The listing builds one solid part. Answer for the finished solid, in the listing's coordinates (mm). A direction names the side the tool comes from. Coordinates: 2 decimals unless noted, no trailing zeros. Order: outer loops, then holes, each group sorted by start corner. A loop starts at its lowest first (then second) coordinate and runs counter-clockwise, first axis right, second up.
```python
from build123d import *

# Parameters (mm, degrees)
CUT_EXTRUDE1_DEPTH = 1.4
SKETCH5_R          = 1.15
CUT_EXTRUDE2_DEPTH = 22.529180779
CUT_EXTRUDE3_DEPTH = 1.475


with BuildPart() as part:
    # Sketch1 → Revolve1 (revolve)
    with BuildSketch(Plane(origin=(0, 0, 0), x_dir=(0, 0, -1), z_dir=(1, 0, 0)), mode=Mode.PRIVATE) as revolve1_sk:
        with BuildLine():
            Line((-1.8375, 0), (1.8375, 0))
            Line((1.8375, 0), (1.8375, 15))
            Line((1.8375, 15), (1.0375, 15))
            Line((1.0375, 15), (1.0375, 14.4))
            ThreePointArc((1.0375, 14.4), (0.3375, 13.7), (-0.3625, 14.4))
            Line((-0.3625, 14.4), (-0.3625, 15))
            Line((-0.3625, 15), (-1.8375, 15))
            Line((-1.8375, 15), (-1.8375, 0))
        make_face()
    revolve(revolve1_sk.sketch.rotate(Axis((0, 0, 1.8375), (0, 0, -1)), 90), axis=Axis((0, 0, 1.8375), (0, 0, -1)))

    # Sketch2 → Cut-Extrude1 (cut)
    with BuildSketch(Plane.XY.offset(1.8375)):
        with BuildLine():
            Line((-2.285166262, 2.846140396), (-14.170034164, 2.196722968))
            ThreePointArc((-14.170034164, 2.196722968), (-16.25, 0), (-14.170034164, -2.196722968))
            Line((-14.170034164, -2.196722968), (-2.285166262, -2.846140396))
            ThreePointArc((-2.285166262, -2.846140396), (3.65, 0), (-2.285166262, 2.846140396))
        make_face()
    extrude(amount=-CUT_EXTRUDE1_DEPTH, mode=Mode.SUBTRACT)

    # Sketch5 → Cut-Extrude2 (cut, through all)
    with BuildSketch(Plane(origin=(0, 0, -1.8375), x_dir=(-1, 0, 0), z_dir=(0, 0, -1))):
        Circle(SKETCH5_R)
    extrude(amount=-CUT_EXTRUDE2_DEPTH, mode=Mode.SUBTRACT)

    # Sketch6 → Cut-Extrude3 (cut)
    with BuildSketch(Plane.XY.offset(0.4375)):
        with BuildLine():
            Line((-14.966629547, -1), (-7, -1))
            Line((-7, -1), (-7, 1))
            Line((-7, 1), (-14.966629547, 1))
            ThreePointArc((-14.966629547, 1), (-14.991655066, 0.500278293), (-15, -5.3e-08))
            ThreePointArc((-15, -5.3e-08), (-14.991655065, -0.500278346), (-14.966629547, -1))
        make_face()
    extrude(amount=-CUT_EXTRUDE3_DEPTH, mode=Mode.SUBTRACT)


solid = part.part
```
(1) For faces 1 (the face through (3.65, -0.11, 1.15)), 2 (the face through (-8, 0, -1.038)), 3 (the face through (-10, -1, 0)), determine the directions among +Z, -Z, +X, -X, +Y, -Y from which every point of the face is accessible in a straight line to the end or side of a thin tool.
(2) Consider line 1 (Y direction, x = 0, z = 1.15); line 2 (Y direction, x = 0, z = -1.3); line 3 (Z direction, x = -6.25, y = 0). Determine where each line is inside the solid, lowest interval first.
(3) Find section B-B (z = 0). Write down the section's boundary in (x, y).
(4) Each of these flat-tipped pins is pushed along its axis until it touches: pin 1 Ø3 at (x, y) = (0, 0) entering from +Z; pin 2 Ø1.2 at (x, z) = (-9, 0) entering from -Y; pin 3 Ø2 at (y, z) = (-4, -0.5) entering from -X. Where does it stop, or does it pass through?
(5) Find section A-A (x = 0). Write down the section's boundary in (y, z), and give its area (3 significant figures).
(6) The mould has two halves that part along Y. Classify faces 4 (the face through (-8.311, -2.517, 1.147)), 5 (the face through (3, 3, 1.838)), 6 (the face through (8.06, -12.65, -1.43)): released by +Y, released by -Y, zero draft, split by the parting line, or undercut.
Findings below:
1. face 1: +Z
1. face 2: none
1. face 3: +Z, -X
2. line 1: y = -15 to -3.65, 3.65 to 15
2. line 2: y = -15 to -1.15, 1.15 to 15
2. line 3: z = -1.84 to 0.44
3. outline: (-13.75, -1) arc R13.79 ccw (long way) to (-13.75, 1) - (-7, 1) - (-7, -1) - close; hole circle Ø2.3 at (0, 0)
4. pin 1: stops at z = 0.44
4. pin 2: stops at y = -12.34
4. pin 3: stops at x = -14.66
5. outline: (-15, -1.84) - (-1.15, -1.84) - (-1.15, 0.44) - (-3.65, 0.44) - (-3.65, 1.84) - (-15, 1.84) - (-15, 0.36) - (-14.4, 0.36) arc R0.7 cw to (-14.4, -1.04) - (-15, -1.04) - close; (1.15, -1.84) - (15, -1.84) - (15, -1.04) - (14.4, -1.04) arc R0.7 cw to (14.4, 0.36) - (15, 0.36) - (15, 1.84) - (3.65, 1.84) - (3.65, 0.44) - (1.15, 0.44) - close
5. area: 91.6 mm2
6. face 4: undercut
6. face 5: zero draft
6. face 6: split by the parting line
